CAD build for the part. Positions are in the model's coordinates, mm. Round coordinates to 2 decimals unless told otherwise and drop trailing zeros. Order: outer loops, then holes, each group sorted by start corner. A loop starts at its lowest first (then second) coordinate and runs counter-clockwise, first axis right, second up. Notation, with made-up numbers: (10.25, 65) - (16.25, 65) arc R10 ccw to (16.25, 77) - close; hole circle Ø3 at (55, 14). An arc over 180 degrees is marked (long way). Write item = value, one per line.
Autodesk Inventor part; units mm, degrees
ref_plane "YZ Plane" through (0, 0, 0) normal (1, 0, 0) x (0, 1, 0)
ref_plane "XZ Plane" through (0, 0, 0) normal (0, 1, 0) x (-1, 0, 0)
ref_plane "XY Plane" through (0, 0, 0) normal (0, 0, 1) x (1, 0, 0)
sketch "Sketch1" plane through (0, 0, 0) normal (1, 0, 0) x (0, 1, 0)
  line L0 (0, 0) -> (76.2, 0)
  line L1 (76.2, 0) -> (76.2, -50.0436)
  line L2 (76.2, -50.0436) -> (0, -50.0436)
  line L3 (0, -50.0436) -> (0, 0)
  arc A0 (26.9905, -50.0436) -> (0, -50.0436) centre (13.4952, -50.0436) ccw
  dimension "d0" = 76.2
extrude "Extrusion1" add sketch "Sketch1" along normal blind 25.4 contours L0 L1 L2 A0 L3
properties part number "holding unit"
(1) Drop a flat-ended pin along its axis: pin 1 (4 mm diameter, centred on x = 20, z = -18, fed in from -Y). Give the stop position or say it passes through.
Solved:
pin_1 = 0
(2) Probe line 1 along Y through (x, z) = (10, -39); line 2 along Y through (x, z) = (9, -42.5); line 3 along Z through (x, y) = (22, 13.5). List the from-to ranges inside material, lowest first.
Solved:
line_1 = 0 to 5.74, 21.25 to 76.2
line_2 = 0 to 2.31, 24.69 to 76.2
line_3 = -36.55 to 0
(3) Band-saw the part on A-A on z = -37.5. List the corners of the cut face in (x, y), plus the area to 3 significant figures.
Solved:
outline = (0, 0) - (25.4, 0) - (25.4, 8.52) - (0, 8.52) - close; (0, 18.47) - (25.4, 18.47) - (25.4, 76.2) - (0, 76.2) - close
area = 1,680 mm²
(4) Pull direction Y, two halves, no side cores. Call faces 1 (the cylindrical face through (12.52, 13.2, -36.55)), 2 (the flat face through (13, 0, -25)), 3 (the flat face through (13, 76.2, -25)), 4 (the flat face through (13, 52, -50.044)): released by +Y, released by -Y, zero draft, split by the parting line, or undercut.
Solved:
face_1 = undercut
face_2 = released by -Y
face_3 = released by +Y
face_4 = zero draft
(5) Band-saw the part on B-B on x = 7. List the corners of the cut face in (y, z).
Solved:
outline = (0, -50.04) arc R13.5 cw to (26.99, -50.04) - (76.2, -50.04) - (76.2, 0) - (0, 0) - close
(6) Band-saw the part on C-C on y = 20.5. List the corners of the cut face in (x, z), plus the area to 3 significant figures.
Solved:
outline = (0, -38.51) - (25.4, -38.51) - (25.4, 0) - (0, 0) - close
area = 978 mm²
